from build123d import *

# Parameters (mm, degrees)
F0_R     = 2.5
F1_DEPTH = 20


with BuildPart() as f1:
    # F0 (on Front) → F1 (new body)
    with BuildSketch(Plane.XZ):
        with BuildLine():
            Line((5, -12.153312), (5, -4.153312))
            ThreePointArc((5, -4.153312), (0, 6.5), (-5, -4.153312))
            Line((-5, -4.153312), (-5, -12.153312))
            Line((-5, -12.153312), (-2.7, -12.153312))
            Line((-2.7, -12.153312), (-2.7, -6.153312))
            Line((-2.7, -6.153312), (2.7, -6.153312))
            Line((2.7, -6.153312), (2.7, -12.153312))
            Line((2.7, -12.153312), (5, -12.153312))
        make_face()
        Circle(F0_R, mode=Mode.SUBTRACT)
    extrude(amount=F1_DEPTH)


solid = f1.part
CAD build for the part. Positions are in the model's coordinates, mm. A direction names the side the tool comes from. Coordinates: 2 decimals unless noted, no trailing zeros. Write each loop counter-clockwise with the first axis right and the second up, starting at its lowest first coordinate (ties: lowest second). Pieces come first, ordered by that corner, then holes. Notation, with made-up numbers: M 15.5,19.5 L 20.5,19.5 A18 ccw 20.5,54.5 Z; hole C 37.5,-14 d1. An arc over 180 degrees is marked long. Return JSON: item names as keys, results as strings.
Item 1: Probe line 1 (Z direction, x = 0, y = -4.75); line 2 (X direction, y = -9, z = -7.5); line 3 (X direction, y = -2.75, z = 0.5). List the from-to ranges inside material, lowest first. Write a range as from..to.
Findings below:
{"line 1": "z = -6.15..-2.5, 2.5..6.5", "line 2": "x = -5..-2.7, 2.7..5", "line 3": "x = -6.48..-2.45, 2.45..6.48"}
Item 2: Drop flat-ended pins along their axis: pin 1 Ø1 at (x, y) = (2, -6) entering from +Z; pin 2 Ø1.8 at (y, z) = (-10, -7.5) entering from +X; pin 3 Ø1.5 at (y, z) = (-8.5, -2) entering from -X; pin 4 Ø1.5 at (x, z) = (-0.5, 0.5) entering from -Y. Give the stop position or say it passes through.
Findings below:
{"pin 1": "stops at z = 6.32", "pin 2": "stops at x = 5", "pin 3": "stops at x = -6.38", "pin 4": "passes through"}
Item 3: Slice it at D-D, the plane z = 5. Write the cut outline in (x, y), and give its area (3 significant figures).
Findings below:
{"outline": "M -4.15,-20 L 4.15,-20 L 4.15,0 L -4.15,0 Z", "area": "166 mm2"}
Item 4: Slice it at A-A, the plane x = 0. Write the cut outline in (y, z), and give its area (3 significant figures).
Findings below:
{"outline": "M -20,-6.15 L 0,-6.15 L 0,-2.5 L -20,-2.5 Z; M -20,2.5 L 0,2.5 L 0,6.5 L -20,6.5 Z", "area": "153 mm2"}
Item 5: Slice it at B-B, the plane z = 0. Write the cut outline in (x, y).
Findings below:
{"outline": "M -6.5,-20 L -2.5,-20 L -2.5,0 L -6.5,0 Z; M 2.5,-20 L 6.5,-20 L 6.5,0 L 2.5,0 Z"}
Item 6: Which spindle directions (+Z, -Z, +X, -X, +Y, -Y) get a long thin tool onto all of the face, cutting with end or side? Do faces 5 (the flat face through (0, 0, -3)), 6 (the flat face through (-5, -10, -8)), 7 (the flat face through (0, -10, -6.153)). Say none if no direction does.
Findings below:
{"face 5": "+Z, -Z, +X, -X, +Y", "face 6": "-Z, -X, +Y, -Y", "face 7": "-Z, +Y, -Y"}
Item 7: Slice it at C-C, the plane y = -4.75. Write the cut outline in (x, z), and give its area (3 significant figures).
Findings below:
{"outline": "M -5,-12.15 L -2.7,-12.15 L -2.7,-6.15 L 2.7,-6.15 L 2.7,-12.15 L 5,-12.15 L 5,-4.15 A6.5 ccw long -5,-4.15 Z; hole C 0,0 d5", "area": "144 mm2"}
Item 8: Two-plate mould, pull along Z, no slides. Class faces 1 (the flat face through (5, -10, -8)), 2 (the cylindrical face through (-0.54, -9.86, -2.44)), 3 (the cylindrical face through (0.206, -9.86, 6.497)), 4 (the flat face through (-4, -10, -12.153)): +Z half, -Z half, draft (parallel to the pull), parting line (faces both ways), or undercut.
Findings below:
{"face 1": "draft", "face 2": "undercut", "face 3": "parting line", "face 4": "-Z half"}
